Can you work these out from the drawing? Everything is in mm from the part's minimum corner. A direction names the side the tool comes from. Round coordinates to 2 decimals unless told otherwise and drop trailing zeros. Loops run counter-clockwise (first coordinate to the right, second up) from the corner with the lowest first, then second, coordinate; pieces in that order, holes last. Notation, with made-up numbers: (18, -16.5) -> (36, -16.5) arc R15 cw to (36, 6.5) -> close; hole circle Ø2 at (-37, 74). An arc over 180 degrees is marked (long way). Answer as a JSON object with one key per item and string values.
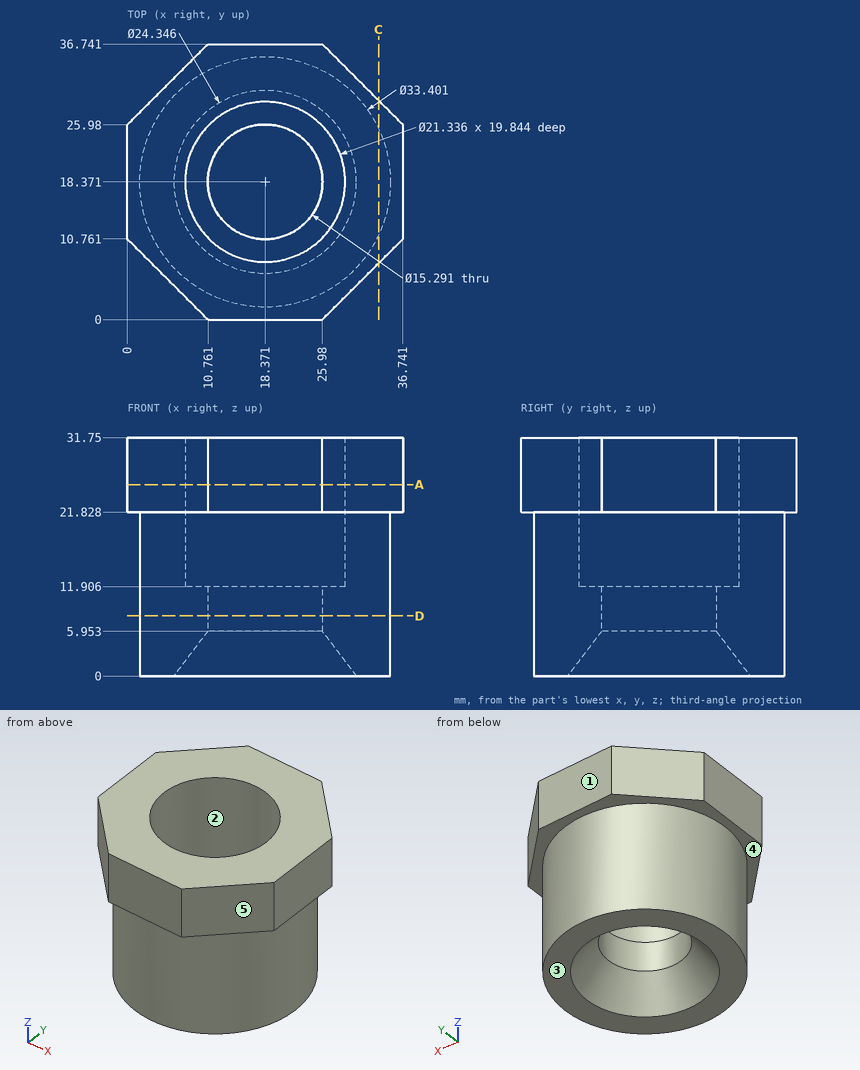
Q1. We'd pull the mould along Y, two halves only. Please class the marked faces 1, 2 and 3: pulls with the +Y half, pulls with the -Y half, needs draft (parallel to the pull), parting line crosses it, or undercut.
Determined:
{"face 1": "pulls with the +Y half", "face 2": "undercut", "face 3": "needs draft"}
Q2. If I drill on L1, parallel to Y at x = 19.5, z = 13.5; L2, parallel to X at y = 24.5, z = 18 (1 decimal); L3, parallel to Z at x = 10.5, y = 34, over which ranges is the centre line in solid material (lowest first)? Write a range as [from, to].
Determined:
{"L1": "[1.71, 7.76], [28.98, 35.03]", "L2": "[2.8, 9.6], [27.1, 33.9]", "L3": "[21.83, 31.75]"}
Q3. I want a section at D-D, the plane z = 8. Write out the boundary of the cut face in (x, y) (1 decimal).
Determined:
{"outline": "circle Ø33.4 at (18.4, 18.4); hole circle Ø15.3 at (18.4, 18.4)"}
Q4. I'm going to push flat-ended pins straight in: pin 1 (10 mm diameter, centred on y = 17, z = 8.5, fed in from +X); pin 2 (8 mm diameter, centred on x = 10, z = 5.5, fed in from +Y); pin 3 (1.5 mm diameter, centred on x = 8.5, z = 16.5, fed in from +Y). Where does each tip first touch, or does it pass through?
Determined:
{"pin 1": "x = 35.07", "pin 2": "y = 34.49", "pin 3": "y = 32.36"}
Q5. I want a section at A-A, the plane z = 25.5. Write out the boundary of the cut face in (x, y).
Determined:
{"outline": "(0, 10.76) -> (10.76, 0) -> (25.98, 0) -> (36.74, 10.76) -> (36.74, 25.98) -> (25.98, 36.74) -> (10.76, 36.74) -> (0, 25.98) -> close; hole circle Ø21.34 at (18.37, 18.37)"}
Q6. I want a section at C-C, the plane x = 33.5. Write out the boundary of the cut face in (y, z), then the cut area to 3 significant figures.
Determined:
{"outline": "(7.52, 21.83) -> (11.3, 21.83) -> (11.3, 0) -> (25.44, 0) -> (25.44, 21.83) -> (29.22, 21.83) -> (29.22, 31.75) -> (7.52, 31.75) -> close", "area": "524 mm²"}
Q7. On a 3-axis mill with a long thin cutter (end or side, diameter ignored), from which of +Z, -Z, +X, -X, +Y, -Y can I reach the whole of each face in a straight line? I mean the marked faces 4 and 5. Say none if no direction works.
Determined:
{"face 4": "-Z", "face 5": "+Z, -Z, +X, -Y"}
